Here's how the part is built. I have some questions about the finished solid (model axes, mm). Coordinates: 2 decimals unless noted, no trailing zeros. Write each loop counter-clockwise with the first axis right and the second up, starting at its lowest first coordinate (ties: lowest second). Pieces come first, ordered by that corner, then holes.
from build123d import *

# Parameters (mm, degrees)
BOSS_EXTRUDE1_DEPTH = 14.986
FILLET1_R           = 2.54
FILLET2_R           = 0.508


with BuildPart() as part:
    # Sketch1 → Revolve1 (revolve)
    with BuildSketch(Plane(origin=(0, 0, 0), x_dir=(0, 0, -1), z_dir=(1, 0, 0)), mode=Mode.PRIVATE) as revolve1_sk:
        with BuildLine():
            Line((-30.226, 0), (-34.544, 0))
            Line((-34.544, 0), (-34.544, 38.1))
            add(Edge.make_bspline(
                [(-34.544, 38.1), (-34.021080338, 40.529206207), (-31.793319074, 41.68897665)],
                knots=[0, 0, 0, 1, 1, 1], degree=2))
            add(Edge.make_bspline(
                [(-31.793319074, 41.68897665), (-17.029892538, 49.760170098), (0, 50.038)],
                knots=[0, 0, 0, 1, 1, 1], degree=2))
            Line((0, 50.038), (0, 44.508100575))
            add(Edge.make_bspline(
                [(-9.398, 42.89990788), (-4.757001601, 44.03505485), (0, 44.508100575)],
                knots=[0, 0, 0, 1, 1, 1], degree=2))
            Line((-9.398, 42.89990788), (-9.398, 45.248349281))
            add(Edge.make_bspline(
                [(-30.226, 38.1), (-23.680294376, 41.89814151), (-16.73762771, 44.280924604), (-9.398, 45.248349281)],
                knots=[0, 0, 0, 0, 0.705520621, 0.705520621, 0.705520621, 0.705520621], degree=3))
            Line((-30.226, 38.1), (-30.226, 0))
        make_face()
    revolve(revolve1_sk.sketch.rotate(Axis((0, 0, 0), (0, 1, 0)), 180), axis=Axis((0, 0, 0), (0, 1, 0)))

    # Sketch2 → Boss-Extrude1 (add)
    with BuildSketch(Plane.XZ):
        with BuildLine():
            ThreePointArc((-3.031237567, 34.410747374), (0.017205772, 35.31933097), (3.064762433, 34.407777714))
            add(Edge.make_bspline(
                [(-3.031237567, 34.410747374), (0.016426392, 33.804246246), (3.064762433, 34.407777714)],
                knots=[0, 0, 0, 1, 1, 1], degree=2))
        make_face()
    extrude(amount=-BOSS_EXTRUDE1_DEPTH)

    # Fillet1
    # the kernel refuses this fillet: 2.54 mm, written as the material it takes off along each edge
    with BuildSketch(Plane(origin=(0.014497608, 14.986, 29.760117923), x_dir=(-0.9885428097510283, 0, -0.15094076086181066), z_dir=(0.15094076086181066, 0, -0.9885428097510283))) as fillet1_piece_1_section:
        with BuildLine():
            CenterArc((5.559213707 - FILLET1_R, -FILLET1_R), FILLET1_R, 0, 90)
            Line((5.559213707 - FILLET1_R, 0), (5.559213707 - FILLET1_R, FILLET1_R * 0.02))
            Line((5.559213707 - FILLET1_R, FILLET1_R * 0.02), (5.559213707 + FILLET1_R * 0.02, FILLET1_R * 0.02))
            Line((5.559213707 + FILLET1_R * 0.02, FILLET1_R * 0.02), (5.559213707 + FILLET1_R * 0.02, -FILLET1_R))
            Line((5.559213707 + FILLET1_R * 0.02, -FILLET1_R), (5.559213707, -FILLET1_R))
        make_face()
    fillet1_piece_1 = revolve(axis=Axis((0.014497608, 14.986, 29.760117923), (0, 1, 0)), revolution_arc=197.418721047, mode=Mode.PRIVATE)
    fillet1_piece_1 = fillet1_piece_1 - Plane(origin=(0, 14.161727142, 0), x_dir=(0, 0, -1), z_dir=(0, 1, 0)) * Cylinder(34.544, 23, mode=Mode.PRIVATE)
    add(fillet1_piece_1, mode=Mode.SUBTRACT)

    # Fillet2
    fillet2_edges = [part.edges().sort_by_distance(p)[0] for p in [
        (0, 0, 30.226),
    ]]
    fillet(fillet2_edges, radius=FILLET2_R)


solid = part.part
1. Thinking about a two-plate mould opening in Z: for faces 1 (the face through (-10.376, 19.317, -32.949)), 2 (the face through (-9.08, 19.04, -28.83)), 3 (the face through (-9.32, 44.09, 1.22)), 4 (the face through (-0.03, 6.14, 35.32)), which applies, pulls with the +Z half, pulls with the -Z half, needs draft (parallel to the pull), parting line crosses it, or undercut?
2. For pin 1 Ø10 at (x, z) = (10, 7.5) entering from +Y; pin 2 Ø6 at (x, y) = (-8, 22.5) entering from +Z; pin 3 Ø10 at (y, z) = (18, -27.5) entering from -X, each with a flat end and sliding along its axis, tell me the tip position at first contact or that it passes through.
3. If I drill on line 1 (X direction, y = 8, z = 0); line 2 (Z direction, x = -7, y = 36); line 3 (Z direction, x = -11.5, y = 34.5), over which ranges is the centre line in solid material (lowest first)?
4. I want a section at A-A (y = 16). List the corners of the cut face in (x, z) for me, then the cut area to 3 significant figures.
Response values:
1. face 1: parting line crosses it
1. face 2: undercut
1. face 3: undercut
1. face 4: pulls with the +Z half
2. pin 1: stops at y = 49.52
2. pin 2: stops at z = 34.18
2. pin 3: stops at x = -26.21
3. line 1: x = -34.54 to -30.23, 30.23 to 34.54
3. line 2: z = -33.83 to -29.4, 29.4 to 33.83
3. line 3: z = -32.57 to -27.95, 27.95 to 32.57
4. outline: circle Ø69.09 at (0, 0); hole circle Ø60.45 at (0, 0)
4. area: 879 mm2
